Geometry check sheet. Reference: the model listing, model coordinates, mm. A direction names the side the tool comes from. Coordinates: 2 decimals unless noted, no trailing zeros. Order: outer loops, then holes, each group sorted by start corner. A loop starts at its lowest first (then second) coordinate and runs counter-clockwise, first axis right, second up. Notation, with made-up numbers: (-37, 48) - (-15, 48) arc R22 ccw to (-15, 73) - close; hole circle Ø6 at (1, 1). An arc over 180 degrees is marked (long way). Return JSON: item names as keys, results as strings. Group by question number.
Item 1: Draft check along Y on faces 1 (the flat face through (-1.268, 13.163, 18.864)), 2 (the cylindrical face through (-50.7, 22.123, 4.516)), 3 (the flat face through (-2.5, 11, 12)), 4 (the flat face through (0, 12, 21)). Enter one of: pulls with the +Y half, pulls with the -Y half, needs draft (parallel to the pull), parting line crosses it, or undercut.
Item 2: Section check B-B on y = 10.75. Enter the section's corners in (x, z), then the cut area to 3 significant figures.
Item 3: Section check D-D on z = 24. Enter the section's corners in (x, y).
Item 4: Gauge pin test, flat ends, axial feed: pin 1 (2 mm diameter, centred on x = -99, z = 14, fed in from +Y); pin 2 (8 mm diameter, centred on y = 16, z = 32, fed in from +X); pin 3 (6 mm diameter, centred on x = -89, y = 18.5, fed in from +Z); pin 4 (8 mm diameter, centred on x = -29.5, y = 21.5, fed in from +Z). Record the tip position at first contact, or that the pin passes through.
Item 5: Scan lines: probe 1 along Y at (x, z) = (-39, 32); probe 2 along X at (y, z) = (3.5, 3); probe 3 along Z at (x, y) = (-9, 12). Record each from-to range of solid material in increasing order.
Item 6: Tool access check on faces 5 (the flat face through (-51, 0, 20)), 6 (the flat face through (-1, 3.044, 16)), 7 (the flat face through (-98.73, 13.16, 18.77)). Record the directions out of +Z, -Z, +X, -X, +Y, -Y that give a thin tool (end or side, any length) a straight path to the whole face; none if there is none.
Item 7: Section check A-A on x = -19. Enter the section's corners in (y, z), then the cut area to 3 significant figures.
Item 8: Section check C-C on z = 20. Enter the section's corners in (x, y).
from build123d import *

# Parameters (mm, degrees)
SKETCH1_W               = 100
SKETCH1_H               = 25
BOSS_EXTRUDE1_DEPTH     = 40
CUT_EXTRUDE2_DEPTH      = 111.566721937
CUT_EXTRUDE2_DEPTH_BACK = 111.566721937
CUT_EXTRUDE3_DEPTH      = 111.566721937
CUT_EXTRUDE3_DEPTH_BACK = 111.566721937
FILLET1_R               = 1
FILLET2_R               = 1
FILLET3_R               = 1
CUT_EXTRUDE5_DEPTH      = 111.566721937
CUT_EXTRUDE5_DEPTH_BACK = 2.5
CUT_EXTRUDE6_DEPTH      = 111.566721937
CUT_EXTRUDE6_DEPTH_BACK = 2.5


with BuildPart() as part:
    # Sketch1 → Boss-Extrude1 (new body)
    with BuildSketch(Plane.XY):
        with Locations((-50, 12.5)):
            Rectangle(SKETCH1_W, SKETCH1_H)
    extrude(amount=BOSS_EXTRUDE1_DEPTH)

    # Sketch2 → Cut-Extrude2 (cut, two sides: drawn at the far end of the back side and taken through both)
    with BuildSketch(Plane(origin=(0, 0, 0), x_dir=(0, 0, -1), z_dir=(1, 0, 0)).offset(-CUT_EXTRUDE2_DEPTH_BACK)):
        Polygon((-121.448428088, -65.214643972), (-40, 0), (-8.776787265, 25), (72.671640823, 90.214643972), (-57.757647122, 253.111500148), (-251.877716033, 97.682212203), align=None)
    extrude(amount=CUT_EXTRUDE2_DEPTH + CUT_EXTRUDE2_DEPTH_BACK, mode=Mode.SUBTRACT)

    # Sketch3 → Cut-Extrude3 (cut, two sides: drawn at the far end of the back side and taken through both)
    with BuildSketch(Plane(origin=(0, 0, 0), x_dir=(0, 0, -1), z_dir=(1, 0, 0)).offset(-CUT_EXTRUDE3_DEPTH_BACK)):
        with BuildLine():
            Line((-62.314729864, 108.995582426), (-7.550030072, 25))
            ThreePointArc((-7.550030072, 25), (-4.293432475, 21.998146007), (0, 20.910491242))
            Line((0, 20.910491242), (100.271779857, 20.929846374))
            Line((100.271779857, 20.929846374), (195.785658883, 197.26707941))
            Line((195.785658883, 197.26707941), (33.199149162, 285.332815462))
            Line((33.199149162, 285.332815462), (-62.314729864, 108.995582426))
        make_face()
    extrude(amount=CUT_EXTRUDE3_DEPTH + CUT_EXTRUDE3_DEPTH_BACK, mode=Mode.SUBTRACT)

    # Fillet1
    fillet1_edges = [part.edges().sort_by_distance(p)[0] for p in [
        (-50, 25, 8.776787265),
    ]]
    fillet(fillet1_edges, radius=FILLET1_R)

    # Fillet2
    fillet2_edges = [part.edges().sort_by_distance(p)[0] for p in [
        (-50, 25, 7.550030072),
    ]]
    fillet(fillet2_edges, radius=FILLET2_R)

    # Fillet3
    fillet3_edges = [part.edges().sort_by_distance(p)[0] for p in [
        (-50, 20.910491242, 0),
    ]]
    fillet(fillet3_edges, radius=FILLET3_R)

    # Sketch4 → Cut-Extrude5 (cut, two sides: drawn at the far end of the back side and taken through both)
    with BuildSketch(Plane(origin=(0, 0, 0), x_dir=(0, 0, -1), z_dir=(1, 0, 0)).offset(-CUT_EXTRUDE5_DEPTH_BACK)):
        Polygon((101.259117222, 3.044212175), (0, 3.044212175), (-30.990460295, 3.044212175), (-6.392305733, 23.56865294), (71.356704641, 88.441607291), (262.495931804, 155.370159656), (292.398344384, 69.97276454), align=None)
    extrude(amount=CUT_EXTRUDE5_DEPTH + CUT_EXTRUDE5_DEPTH_BACK, mode=Mode.SUBTRACT)

    # Sketch5 → Cut-Extrude6 (cut, two sides: drawn at the far end of the back side and taken through both)
    with BuildSketch(Plane.ZY.offset(100).offset(-CUT_EXTRUDE6_DEPTH_BACK)):
        Polygon((-101.259117222, 3.044212175), (0, 3.044212175), (30.8250701, 3.044212175), (6.37948349, 23.555780442), (-71.190616863, 88.642555993), (-262.263101068, 155.761413714), (-292.331601426, 70.163069896), align=None)
    extrude(amount=CUT_EXTRUDE6_DEPTH + CUT_EXTRUDE6_DEPTH_BACK, mode=Mode.SUBTRACT)


solid = part.part
Computed:
{
 "1": {"face 1": "undercut", "face 2": "pulls with the +Y half", "face 3": "undercut", "face 4": "needs draft"},
 "2": {"outline": "(-100, 21.64) - (-97.5, 21.64) - (-97.5, 0) - (-2.5, 0) - (-2.5, 21.76) - (0, 21.76) - (0, 26.57) - (-100, 26.57) - close", "area": "2,550 mm²"},
 "3": {"outline": "(-100, 0) - (0, 0) - (0, 3.04) - (-2.5, 3.04) - (-2.5, 8.88) - (0, 8.88) - (0, 12.81) - (-100, 12.81) - (-100, 8.77) - (-97.5, 8.77) - (-97.5, 3.04) - (-100, 3.04) - close"},
 "4": {"pin 1": "stops at y = 21.62", "pin 2": "passes through", "pin 3": "stops at z = 20.64", "pin 4": "stops at z = 18.14"},
 "5": {"probe 1": "y = 0 to 6.41", "probe 2": "x = -97.5 to -2.5", "probe 3": "z = 0 to 25.01"},
 "6": {"face 5": "+Z, -Z, +X, -X, -Y", "face 6": "-Z, +X", "face 7": "-Z, -X"},
 "7": {"outline": "(0, 0) - (19.96, 0) arc R1 ccw to (20.96, 0.9) arc R9.01 cw to (24.59, 7.27) arc R1 ccw to (25, 8.07) - (25, 8.43) arc R1 ccw to (24.78, 9.05) - (0, 40) - close", "area": "588 mm²"},
 "8": {"outline": "(-100, 0) - (0, 0) - (0, 3.04) - (-2.5, 3.04) - (-2.5, 12.21) - (0, 12.21) - (0, 16.01) - (-100, 16.01) - (-100, 12.13) - (-97.5, 12.13) - (-97.5, 3.04) - (-100, 3.04) - close"}
}
